CAD build for the part. Positions are in the model's coordinates, mm. Face numbers are marked on the shaded views. Round coordinates to 2 decimals unless told otherwise and drop trailing zeros. Loops run counter-clockwise (first coordinate to the right, second up) from the corner with the lowest first, then second, coordinate; pieces in that order, holes last.
from build123d import *

# Parameters (mm, degrees)
EXTRUDE_SKETCH003_DEPTH = 6.5
POCKET001_DEPTH         = 5
FILLET002_R             = 1


with BuildPart() as part:
    # Sketch003 → Extrude_Sketch003 (new body)
    with BuildSketch(Plane(origin=(0, 0, 0), x_dir=(0, -1, 0), z_dir=(-1, 0, 0))):
        Polygon((-17, 5), (-9, 5), (-10, 1.5), (-16, 1.5), align=None)
    extrude(amount=-EXTRUDE_SKETCH003_DEPTH)

    # Sketch004 → Pocket001 (cut)
    with BuildSketch(Plane(origin=(0, 0, 0), x_dir=(0, -1, 0), z_dir=(-1, 0, 0))):
        Polygon((-15.632888, 4.295265), (-10.592995, 4.295265), (-11.18045, 2.239173), (-15.045433, 2.239173), align=None)
    extrude(amount=-POCKET001_DEPTH, mode=Mode.SUBTRACT)

    # Fillet002
    fillet002_edges = [part.edges().sort_by_distance(p)[0] for p in [
        (3.25, 17, 5),
        (3.25, 9, 5),
    ]]
    fillet(fillet002_edges, radius=FILLET002_R)


solid = part.part
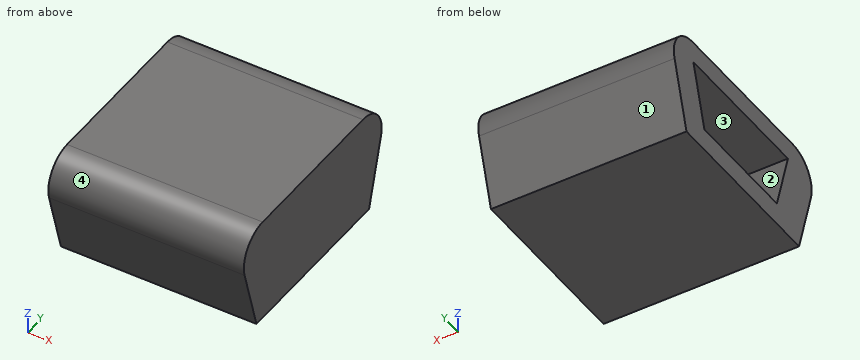
Item 1: Cut at D-D (z = 2.4). List the corners of the cut face in (x, y).
Verdict:
outline: (0, 9.74) - (6.5, 9.74) - (6.5, 16.26) - (0, 16.26) - (0, 15.09) - (5, 15.09) - (5, 11.13) - (0, 11.13) - close
Item 2: Cut at C-C (x = 6). List the corners of the cut face in (y, z).
Verdict:
outline: (9.36, 3.73) - (10, 1.5) - (16, 1.5) - (16.64, 3.73) arc R1 ccw to (15.67, 5) - (10.33, 5) arc R1 ccw to start
Item 3: Mould opens along Y. For the marked faces 1, 2, 3 and 4 say: released by +Y, released by -Y, zero draft, split by the parting line, or undercut.
Verdict:
face 1: released by +Y
face 2: undercut
face 3: undercut
face 4: released by -Y
Item 4: Cut at A-A (x = 1.5). List the corners of the cut face in (y, z), plus the area to 3 significant figures.
Verdict:
outline: (9.36, 3.73) - (10, 1.5) - (16, 1.5) - (16.64, 3.73) arc R1 ccw to (15.67, 5) - (10.33, 5) arc R1 ccw to start; hole (10.59, 4.3) - (11.18, 2.24) - (15.05, 2.24) - (15.63, 4.3) - close
area: 14.5 mm2
Item 5: Wall check: L1, parallel to Z at x = 1.75, y = 13.5; L2, parallel to X at y = 12.5, z = 4.15; L3, parallel to Y at x = 4.5, z = 2.4. Give the ranges that are in metal, low to high.
Verdict:
L1: z = 1.5 to 2.24, 4.3 to 5
L2: x = 5 to 6.5
L3: y = 9.74 to 11.13, 15.09 to 16.26
Item 6: Cut at B-B (y = 14.75). List the corners of the cut face in (x, z), plus the area to 3 significant figures.
Verdict:
outline: (0, 1.5) - (6.5, 1.5) - (6.5, 5) - (0, 5) - (0, 4.3) - (5, 4.3) - (5, 2.24) - (0, 2.24) - close
area: 12.5 mm2
